Input: part model. Units: mm. Frame: model coordinates. Face numbers are marked on the shaded views. A direction names the side the tool comes from. Coordinates: 2 decimals unless noted, no trailing zeros. Order: outer loops, then holes, each group sorted by start corner. A loop starts at its lowest first (then second) coordinate and runs counter-clockwise, first axis right, second up. Notation, with made-up numbers: (33, -11) - (69, -11) arc R20 cw to (69, -1) - close; hole circle Ø3 at (84.25, 42). An arc over 180 degrees is marked (long way). Answer as CSV lines item,"result". Start each with the question number.
Item 1: Section B-B (y = -6). Output: boundary loops of the cut face in (x, z).
Item 2: Draft query along X for the marked faces 1, 2, 3 and 4. Return one class per face: +X half, -X half, draft (parallel to the pull), parting line (faces both ways), or undercut.
Item 3: Access query for the marked faces 5 and 6. Directions: +Z, -Z, +X, -X, +Y, -Y. A direction counts if a zero-diameter tool reaches every point of the face in a straight line with its end or side. Return the directions, or none.
Item 4: First-contact query: pin 1 (1 mm diameter, centred on x = -23.5, z = 16.5, fed in from -Y); pin 2 (1.5 mm diameter, centred on x = -23, y = -9, fed in from -Z); pin 3 (1.5 mm diameter, centred on x = -24.5, y = -5.5, fed in from +Z). Flat tips, straight axial feed; report the tip coordinate or a pass-through.
Item 5: Material intervals for line 1 along Y through (x, z) = (-19.5, 15.25); line 2 along Z through (x, y) = (-19.5, -5.5); line 3 along Z through (x, y) = (-19, -1.25), sorted ascending.
Item 6: Section A-A (x = -24). Output: boundary loops of the cut face in (y, z), and give its area (3 significant figures).
Item 7: Section D-D (x = -19). Output: boundary loops of the cut face in (y, z), and give its area (3 significant figures).
Item 8: Section C-C (z = 9.25). Output: boundary loops of the cut face in (x, y), and give its area (3 significant figures).
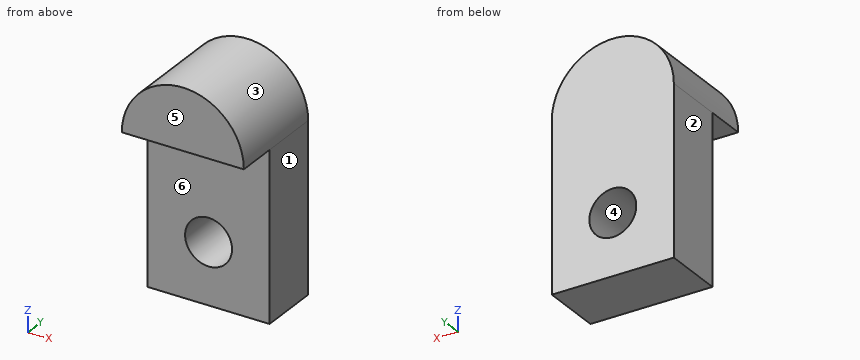
from build123d import *

# Parameters (mm, degrees)
F0_W     = 15.24
F0_H     = 20.9549992294
F0_R     = 2.9310682444
F1_DEPTH = 7.62
F2_DEPTH = 12.7


with BuildPart() as f1:
    # F0 (on Front) → F1 (new body)
    with BuildSketch(Plane.XZ):
        with BuildLine():
            ThreePointArc((-13.9654323469, 25.8065824842), (-21.5854323469, 33.4265824842), (-29.2054323469, 25.8065824842))
            Line((-29.2054323469, 25.8065824842), (-13.9654323469, 25.8065824842))
        make_face()
        with Locations((-21.5854323469, 15.3290828695)):
            Rectangle(F0_W, F0_H)
        with Locations((-21.5854323469, 12.4715832548)):
            Circle(F0_R, mode=Mode.SUBTRACT)
    extrude(amount=F1_DEPTH)

    # F0 (on Front) → F2 (join)
    with BuildSketch(Plane.XZ):
        with BuildLine():
            ThreePointArc((-13.9654323469, 25.8065824842), (-21.5854323469, 33.4265824842), (-29.2054323469, 25.8065824842))
            Line((-29.2054323469, 25.8065824842), (-13.9654323469, 25.8065824842))
        make_face()
    extrude(amount=F2_DEPTH)


solid = f1.part
Determined:
1,outline,"(-29.21, 4.85) - (-13.97, 4.85) - (-13.97, 25.81) arc R7.62 ccw to (-29.21, 25.81) - close; hole circle Ø5.86 at (-21.59, 12.47)"
2,face 1,"+X half"
2,face 2,"-X half"
2,face 3,"parting line"
2,face 4,"undercut"
3,face 5,"+Z, -Z, +X, -X, -Y"
3,face 6,"-Z, +X, -X, -Y"
4,pin 1,"stops at y = -7.62"
4,pin 2,"stops at z = 25.81"
4,pin 3,"stops at z = 33.11"
5,line 1,"y = -7.62 to 0"
5,line 2,"z = 4.85 to 10.41, 14.53 to 33.14"
5,line 3,"z = 4.85 to 11.09, 13.85 to 32.97"
6,outline,"(-12.7, 25.81) - (-7.62, 25.81) - (-7.62, 14.13) - (0, 14.13) - (0, 33.03) - (-12.7, 33.03) - close; (-7.62, 4.85) - (0, 4.85) - (0, 10.81) - (-7.62, 10.81) - close"
6,area,"226 mm^2"
7,outline,"(-12.7, 25.81) - (-7.62, 25.81) - (-7.62, 13.85) - (0, 13.85) - (0, 32.97) - (-12.7, 32.97) - close; (-7.62, 4.85) - (0, 4.85) - (0, 11.09) - (-7.62, 11.09) - close"
7,area,"230 mm^2"
8,outline,"(-29.21, -7.62) - (-13.97, -7.62) - (-13.97, 0) - (-29.21, 0) - close"
8,area,"116 mm^2"
